```python
from build123d import *

# Parameters (mm, degrees)
SKETCH2_R               = 2.25
BOSS_EXTRUDE1_DEPTH     = 10
CUT_EXTRUDE_THIN1_START = -3
SKETCH3_R               = 104
SKETCH3_R_2             = 4
CUT_EXTRUDE_THIN1_DEPTH = 3
SKETCH4_R               = 104
SKETCH4_R_2             = 4
CUT_EXTRUDE_THIN2_DEPTH = 3


with BuildPart() as part:
    # Sketch2 → Boss-Extrude1 (new body)
    with BuildSketch(Plane.XY):
        with BuildLine():
            Line((0, 4), (92.1, 4))
            ThreePointArc((92.1, 4), (96.1, 0), (92.1, -4))
            Line((92.1, -4), (0, -4))
            ThreePointArc((0, -4), (-4, 0), (0, 4))
        make_face()
        Circle(SKETCH2_R, mode=Mode.SUBTRACT)
        with Locations((92.1, 0)):
            Circle(SKETCH2_R, mode=Mode.SUBTRACT)
    extrude(amount=BOSS_EXTRUDE1_DEPTH)

    # Sketch3 → Cut-Extrude-Thin1 (cut)
    with BuildSketch(Plane.XY.offset(10).offset(CUT_EXTRUDE_THIN1_START)):
        Circle(SKETCH3_R)
        Circle(SKETCH3_R_2, mode=Mode.SUBTRACT)
    extrude(amount=CUT_EXTRUDE_THIN1_DEPTH, mode=Mode.SUBTRACT)

    # Sketch4 → Cut-Extrude-Thin2 (cut)
    with BuildSketch(Plane(origin=(0, 0, 0), x_dir=(-1, 0, 0), z_dir=(0, 0, -1))):
        with Locations((-92.1, 0)):
            Circle(SKETCH4_R)
        with Locations((-92.1, 0)):
            Circle(SKETCH4_R_2, mode=Mode.SUBTRACT)
    extrude(amount=-CUT_EXTRUDE_THIN2_DEPTH, mode=Mode.SUBTRACT)


solid = part.part
```
Source: CAD feature listing. Evaluate the final solid. Frame: model axes, mm. Round coordinates to 2 decimals unless told otherwise and drop trailing zeros. Loops run counter-clockwise (first coordinate to the right, second up) from the corner with the lowest first, then second, coordinate; pieces in that order, holes last. Notation, with made-up numbers: M 88,33.5 L 92,33.5 A17 cw 92,56.5 Z; hole C 46.5,68.25 d6. An arc over 180 degrees is marked long. Use a Markdown table: item, result. Add a question column.
1. Section query A-A on z = 4.5. Return the cut outline in (x, y).
2. Mould query, pull axis X, two halves, no side actions, for faces 1 (the cylindrical face through (96.096, 0.176, 2.673)), 2 (the flat face through (45, 0, 3)), 3 (the cylindrical face through (-0.29, 2.23, 6.45)). Classes: pulls with the +X half, pulls with the -X half, needs draft (parallel to the pull), parting line crosses it, or undercut.
3. Section query B-B on y = 1.25. Return the cut outline in (x, z), then the cut area to 3 significant figures.
4. Section query D-D on x = 50. Return the cut outline in (y, z), then the cut area to 3 significant figures.
5. Section query C-C on z = 8.5. Return the cut outline in (x, y), then the cut area to 3 significant figures.
6. Line query: line 1 (X direction, y = 0, z = 6); line 2 (X direction, y = 0, z = 7.5); line 3 (X direction, y = -1.75, z = 4). Output: solid intervals per line, ascending.
7. Contact query for flat-ended pins moving along their axis: P1, Ø4, axis at x = 53, y = 0.5, coming from the -Z side; P2, Ø2, axis at x = 8.5, y = -2.5, coming from the +Z side. Output: stop coordinate, or through.
Reported:
| question | item | result |
|---|---|---|
| 1 | outline | M 0,-4 L 92.1,-4 A4 ccw 92.1,4 L 0,4 A4 ccw Z; hole C 0,0 d4.5; hole C 92.1,0 d4.5 |
| 2 | face 1 | parting line crosses it |
| 2 | face 2 | needs draft |
| 2 | face 3 | undercut |
| 3 | outline | M -3.8,3 L -1.87,3 L -1.87,10 L -3.8,10 Z; M 1.87,3 L 88.3,3 L 88.3,0 L 90.23,0 L 90.23,7 L 3.8,7 L 3.8,10 L 1.87,10 Z; M 93.97,0 L 95.9,0 L 95.9,7 L 93.97,7 Z |
| 3 | area | 392 mm² |
| 4 | outline | M -4,3 L 4,3 L 4,7 L -4,7 Z |
| 4 | area | 32.0 mm² |
| 5 | outline | C 0,0 d8; hole C 0,0 d4.5 |
| 5 | area | 34.4 mm² |
| 6 | line 1 | x = -4 to -2.25, 2.25 to 89.85, 94.35 to 96.1 |
| 6 | line 2 | x = -4 to -2.25, 2.25 to 4 |
| 6 | line 3 | x = -3.6 to -1.41, 1.41 to 90.69, 93.51 to 95.7 |
| 7 | P1 | stops at z = 3 |
| 7 | P2 | stops at z = 7 |
